Work out the finished part from the listing and answer in its coordinate system (mm). Give positions to 0.01 mm unless a question says otherwise; leave off trailing zeros. Loops run counter-clockwise (first coordinate to the right, second up) from the corner with the lowest first, then second, coordinate; pieces in that order, holes last.
from build123d import *

# Parameters (mm, degrees)
F0_R     = 60.541459453
F2_DEPTH = 3.175


# Not quite as in the source:
# - the program builds the solid bodies; features that only make, move or delete a surface that nothing else refers to are left out


with BuildPart() as f2:
    # F0 (on Top) → F2 (new body, symmetric)
    with BuildSketch(Plane.XY):
        with BuildLine():
            ThreePointArc((29.63795994, 120.4253280383), (0, 107.6024649325), (-29.63795994, 120.4253280383))
            ThreePointArc((-29.63795994, 120.4253280383), (-31.4004725935, 122.4295872496), (-33.0277066154, 124.5451522517))
            ThreePointArc((-33.0277066154, 124.5451522517), (-136.833025163, 119.6500101861), (-110.5775391502, 19.1007385387))
            ThreePointArc((-110.5775391502, 19.1007385387), (-102.1103333636, 0), (-110.5775391502, -19.1007385387))
            ThreePointArc((-110.5775391502, -19.1007385387), (-136.833025163, -119.6500101861), (-33.0277066154, -124.5451522517))
            ThreePointArc((-33.0277066154, -124.5451522517), (-31.4004725935, -122.4295872496), (-29.63795994, -120.4253280383))
            ThreePointArc((-29.63795994, -120.4253280383), (0, -107.6024649325), (29.63795994, -120.4253280383))
            ThreePointArc((29.63795994, -120.4253280383), (135.2096998467, -121.7674331009), (110.5775391502, -19.1007385387))
            ThreePointArc((110.5775391502, -19.1007385387), (102.1103333636, 0), (110.5775391502, 19.1007385387))
            ThreePointArc((110.5775391502, 19.1007385387), (135.2096998467, 121.7674331009), (29.63795994, 120.4253280383))
        make_face()
        with Locations((-82.9460425302, -80.0184514167)):
            Circle(F0_R, mode=Mode.SUBTRACT)
        with Locations((82.9460425302, -80.0184514167)):
            Circle(F0_R, mode=Mode.SUBTRACT)
        with BuildLine():
            add(Edge.make_bspline(
                [(0, -76.0996581864), (9.5787021029, -69.2053000853), (33.1312215182, -54.3582389446), (31.8321399477, 37.4809793102), (0, 80.0184514167)],
                knots=[0, 0, 0, 0, 0.3369505381, 1, 1, 1, 1], degree=3))
            add(Edge.make_bspline(
                [(0, -76.0996581864), (-9.5787021029, -69.2053000853), (-33.1312215182, -54.3582389446), (-31.8321399477, 37.4809793102), (0, 80.0184514167)],
                knots=[0, 0, 0, 0, 0.3369505381, 1, 1, 1, 1], degree=3))
        make_face(mode=Mode.SUBTRACT)
        with Locations((-82.9460425302, 80.0184514167)):
            Circle(F0_R, mode=Mode.SUBTRACT)
        with Locations((82.9460425302, 80.0184514167)):
            Circle(F0_R, mode=Mode.SUBTRACT)
    extrude(amount=F2_DEPTH, both=True)


solid = f2.part
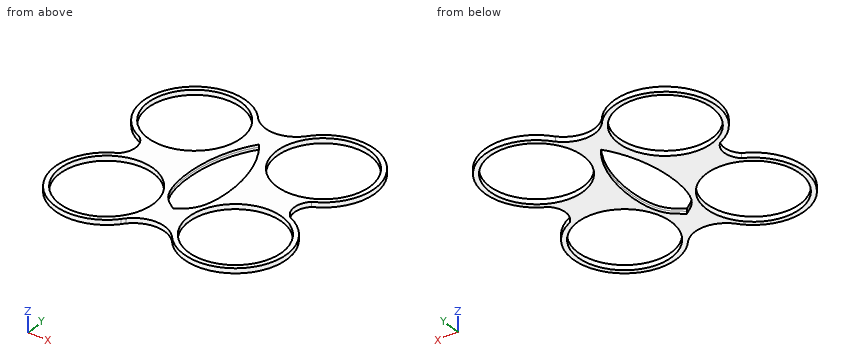
Item 1: Find section D-D, the plane z = 1.5. Give the number of separate pieces and of enclosed holes in the cut face, plus the area to 3 significant figures.
Item 2: A flat-ended cylindrical pin translates along its axis: pin 1 Ø1 at (x, z) = (-73.5, -1) entering from -Y. Find the tip coordinate at first contact, or state that the pin passes through.
Item 3: Find section A-A, the plane x = 51.5. Write down the section's boundary in (y, z) (3 decimals), plus the area to 3 significant figures.
Item 4: Consider line 1 (X direction, y = -82, z = 2.25); line 2 (X direction, y = 133, z = -2.5); line 3 (X direction, y = 94, z = 2.75). Determine where each line is inside the solid, lowest interval first.
Item 5: Find section B-B, the plane y = 114. Write down the section's boundary in (x, z) (3 decimals).
Item 6: Find section C-C, the plane x = -129. Write down the section's boundary in (y, z) (3 decimals), plus the area to 3 significant figures.
Ans:
1. separate pieces: 1
1. enclosed holes: 5
1. area: 19,800 mm2
2. pin 1: stops at y = -146.31
3. outline: (-139.058, -3.175) - (-131.753, -3.175) - (-131.753, 3.175) - (-139.058, 3.175) - close; (-28.284, -3.175) - (28.284, -3.175) - (28.284, 3.175) - (-28.284, 3.175) - close; (131.753, -3.175) - (139.058, -3.175) - (139.058, 3.175) - (131.753, 3.175) - close
3. area: 452 mm2
4. line 1: x = -149.81 to -143.46, -22.44 to 22.44, 143.46 to 149.81
4. line 2: x = -123.78 to -112.24, -53.65 to -42.11, 42.11 to 53.65, 112.24 to 123.78
4. line 3: x = -148.36 to -141.85, -24.04 to 24.04, 141.85 to 148.36
5. outline: (-140.563, -3.175) - (-133.051, -3.175) - (-133.051, 3.175) - (-140.563, 3.175) - close; (-32.841, -3.175) - (-21.894, -3.175) - (-21.894, 3.175) - (-32.841, 3.175) - close; (21.894, -3.175) - (32.841, -3.175) - (32.841, 3.175) - (21.894, 3.175) - close; (133.051, -3.175) - (140.563, -3.175) - (140.563, 3.175) - (133.051, 3.175) - close
6. outline: (-128.531, -3.175) - (-119.316, -3.175) - (-119.316, 3.175) - (-128.531, 3.175) - close; (-40.721, -3.175) - (-31.506, -3.175) - (-31.506, 3.175) - (-40.721, 3.175) - close; (31.506, -3.175) - (40.721, -3.175) - (40.721, 3.175) - (31.506, 3.175) - close; (119.316, -3.175) - (128.531, -3.175) - (128.531, 3.175) - (119.316, 3.175) - close
6. area: 234 mm2
